```python
from build123d import *

# Parameters (mm, degrees)
SKETCH1_W           = 250
SKETCH1_H           = 250
SKETCH1_W_2         = 230
SKETCH1_H_2         = 230
BOSS_EXTRUDE1_DEPTH = 90
SKETCH2_W           = 200
SKETCH2_H           = 70
CUT_EXTRUDE1_DEPTH  = 50
FILLET1_R           = 20
BOSS_EXTRUDE2_DEPTH = 25
BOSS_EXTRUDE3_DEPTH = 25
SKETCH6_W           = 190
SKETCH6_H           = 30
CUT_EXTRUDE2_DEPTH  = 251


with BuildPart() as part:
    # Sketch1 → Boss-Extrude1 (new body)
    with BuildSketch(Plane(origin=(0, 0, 0), x_dir=(1, 0, 0), z_dir=(0, 1, 0))):
        Rectangle(SKETCH1_W, SKETCH1_H)
        Rectangle(SKETCH1_W_2, SKETCH1_H_2, mode=Mode.SUBTRACT)
    extrude(amount=BOSS_EXTRUDE1_DEPTH)

    # Sketch2 → Cut-Extrude1 (cut)
    with BuildSketch(Plane.XY.offset(125)):
        with Locations((0, 35)):
            Rectangle(SKETCH2_W, SKETCH2_H)
    extrude(amount=-CUT_EXTRUDE1_DEPTH, mode=Mode.SUBTRACT)

    # Fillet1
    fillet1_edges = [part.edges().sort_by_distance(p)[0] for p in [
        (-115, 45, 115),
        (115, 45, 115),
        (115, 45, -115),
        (-115, 45, -115),
        (-125, 45, 125),
        (125, 45, 125),
        (125, 45, -125),
        (-125, 45, -125),
    ]]
    fillet(fillet1_edges, radius=FILLET1_R)

    # Sketch4 → Boss-Extrude2 (add, symmetric)
    with BuildSketch(Plane.XY):
        Polygon((-115, 45), (-90, 45), (-115, 20), align=None)
        Polygon((115, 45), (90, 45), (115, 20), align=None)
    extrude(amount=BOSS_EXTRUDE2_DEPTH, both=True)

    # Sketch5 → Boss-Extrude3 (add, symmetric)
    with BuildSketch(Plane(origin=(0, 0, 0), x_dir=(0, 0, -1), z_dir=(1, 0, 0))):
        Polygon((115, 45), (115, 20), (90, 45), align=None)
    extrude(amount=BOSS_EXTRUDE3_DEPTH, both=True)

    # Sketch6 → Cut-Extrude2 (cut, through all)
    with BuildSketch(Plane(origin=(125, 0, 0), x_dir=(0, 0, -1), z_dir=(1, 0, 0))):
        with Locations((0, 15)):
            Rectangle(SKETCH6_W, SKETCH6_H)
    extrude(amount=-CUT_EXTRUDE2_DEPTH, mode=Mode.SUBTRACT)


solid = part.part
```
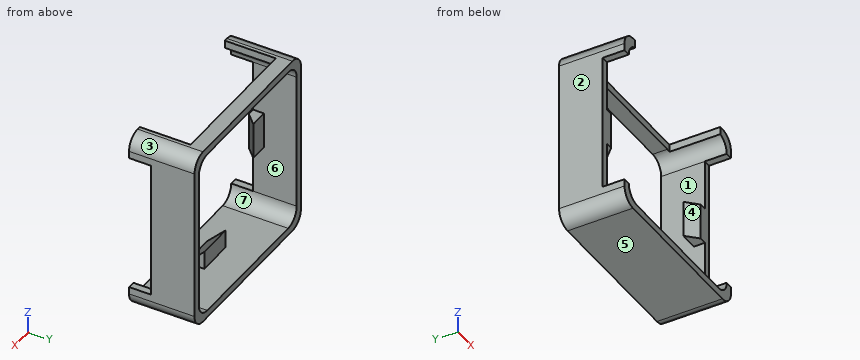
For this review, take the finished solid that the model builds, in its own axes (mm). Face numbers are marked on the shaded views. A direction names the side the tool comes from. Give positions to 0.01 mm unless a question says otherwise; leave off trailing zeros. Write each loop counter-clockwise with the first axis right and the second up, starting at its lowest first coordinate (ties: lowest second). Pieces come first, ordered by that corner, then holes.
Item 1: Machinability: for the marked faces 4, 5, 6 and 7, which of the approach directions +Z, -Z, +X, -X, +Y, -Y give a long, thin tool a straight path to every point of the face, cutting with its end or side? Answer none if there is none.
Item 2: The part is to be moulded in two halves that separate along Z. For the marked faces 1, 2 and 3, say which applies: +Z half, -Z half, draft (parallel to the pull), parting line (faces both ways), or undercut.
Item 3: Wall thickness on probe 1 along X at (y, z) = (70, 71); probe 2 along Z at (x, y) = (-7, 52): over which ranges is each line inside the solid? List them lowest first.
Item 4: Take a section at A-A (z = -67.5). Give the boundary of the cut face in (x, y), and give its area (3 significant figures).
Item 5: Take a section at C-C (y = 9). Give the boundary of the cut face in (x, z), and give its area (3 significant figures).
Item 6: Take a section at D-D (z = -98). Give the boundary of the cut face in (x, y).
Item 7: Take a section at B-B (x = 13). Give the boundary of the cut face in (y, z).
Item 8: Insertion check: P1, Ø5, axis at x = -84.5, y = 20, coming from the +Z side; P2, Ø11.5, axis at y = 31, z = 121.5, coming from the -X side; P3, Ø11.5, axis at y = 26, z = 120.5, coming from the +X side. Each pin has a flat end and moves straight along its axis. Give the tip position at first contact, or say it passes through.
Established:
1. face 4: -Y
1. face 5: -Z, +X, -X, +Y, -Y
1. face 6: +Y
1. face 7: +Y, -Y
2. face 1: undercut
2. face 2: draft
2. face 3: +Z half
3. probe 1: x = -125 to -115, 115 to 125
3. probe 2: z = -125 to -115
4. outline: (-125, 30) - (-115, 30) - (-115, 90) - (-125, 90) - close; (115, 30) - (125, 30) - (125, 90) - (115, 90) - close
4. area: 1,200 mm2
5. outline: (-125, -105) arc R20 ccw to (-105, -125) - (105, -125) arc R20 ccw to (125, -105) - (125, -95) - (115, -95) arc R20 cw to (95, -115) - (-95, -115) arc R20 cw to (-115, -95) - (-125, -95) - close; (-125, 95) - (-115, 95) arc R20 cw to (-100, 114.36) - (-100, 125) - (-105, 125) arc R20 ccw to (-125, 105) - close; (100, 114.36) arc R20 cw to (115, 95) - (125, 95) - (125, 105) arc R20 ccw to (105, 125) - (100, 125) - close
5. area: 3,800 mm2
6. outline: (-125, 0) - (-114.77, 0) - (-114.77, 90) - (-125, 90) - close; (-25, 37) - (25, 37) - (25, 45) - (-25, 45) - close; (114.77, 0) - (125, 0) - (125, 90) - (114.77, 90) - close
7. outline: (0, -125) - (90, -125) - (90, -115) - (45, -115) - (45, -90) - (20, -115) - (0, -115) - close; (70, 115) - (90, 115) - (90, 125) - (70, 125) - close
8. P1: stops at z = -115
8. P2: stops at x = -121.87
8. P3: stops at x = 122.46
